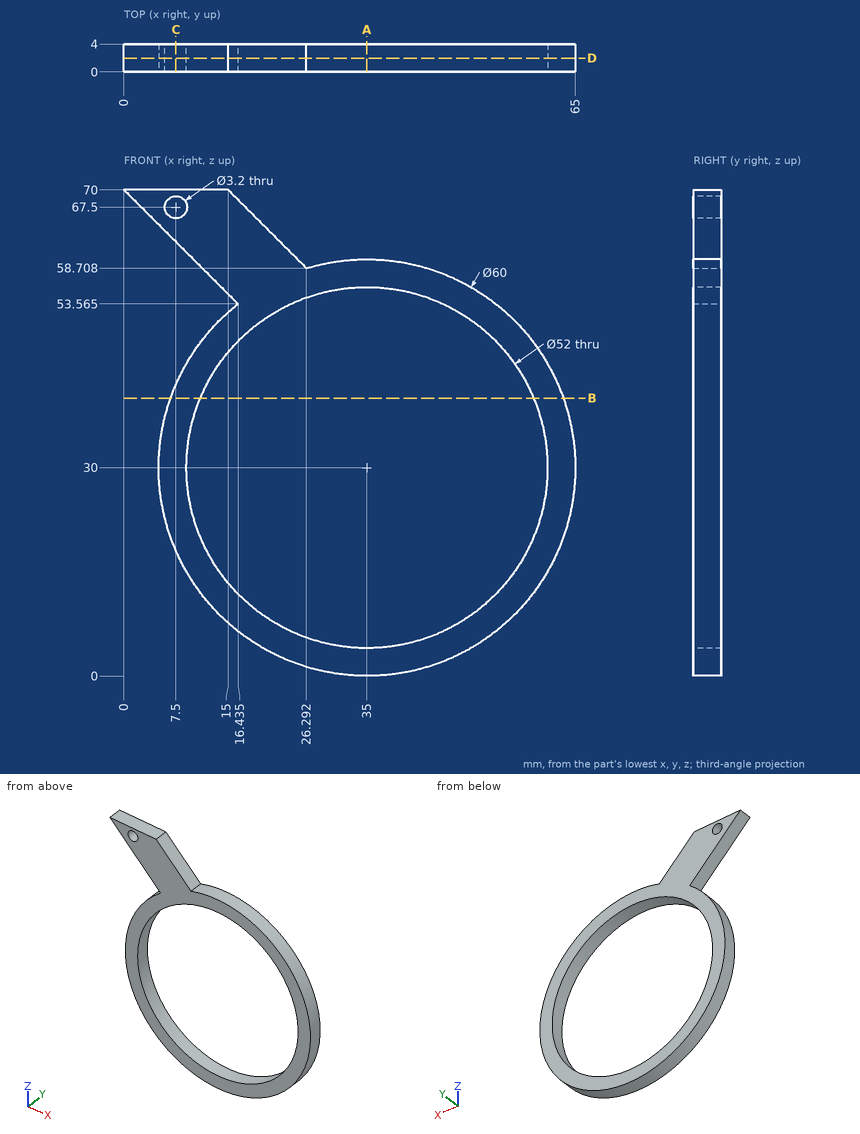
Part print with two shaded views. Sizes in mm from the minimum x, y, z corner. Give positions to 0.01 mm unless a question says otherwise; leave off trailing zeros. Write each loop counter-clockwise with the first axis right and the second up, starting at its lowest first coordinate (ties: lowest second). Pieces come first, ordered by that corner, then holes.
1) Cut at C-C on x = 7.5. Write the cut outline in (y, z).
Resolved:
outline: (0, 18.01) - (4, 18.01) - (4, 41.99) - (0, 41.99) - close; (0, 62.5) - (4, 62.5) - (4, 65.9) - (0, 65.9) - close; (0, 69.1) - (4, 69.1) - (4, 70) - (0, 70) - close
2) Pin check, flat tip, straight feed: pin 1 (1 mm diameter, centred on y = 2.5, z = 55.5, fed in from +X) (1 decimal). Stop position of the tip, or through.
Resolved:
pin 1: stops at x = 51.6
3) Cut at B-B on z = 40. Write the cut outline in (x, y) (1 decimal).
Resolved:
outline: (6.7, 0) - (11, 0) - (11, 4) - (6.7, 4) - close; (59, 0) - (63.3, 0) - (63.3, 4) - (59, 4) - close
4) Probe L1, parallel to Z at x = 35, y = 1; L2, parallel to Z at x = 7.5, y = 1.1 (1 decimal); L3, parallel to X at y = 0.6, z = 29.5 (1 decimal). List the from-to ranges inside material, lowest first.
Resolved:
L1: z = 0 to 4, 56 to 60
L2: z = 18 to 42, 62.5 to 65.9, 69.1 to 70
L3: x = 5 to 9, 61 to 65
5) Cut at A-A on x = 35. Write the cut outline in (y, z).
Resolved:
outline: (0, 0) - (4, 0) - (4, 4) - (0, 4) - close; (0, 56) - (4, 56) - (4, 60) - (0, 60) - close
6) Cut at D-D on y = 1.95. Write the cut outline in (x, z) (1 decimal).
Resolved:
outline: (0, 70) - (16.4, 53.6) arc R30 ccw (long way) to (26.3, 58.7) - (15, 70) - close; hole circle Ø3.2 at (7.5, 67.5); hole circle Ø52 at (35, 30)
